Verification items for the finished model (mm, model axes). Face numbers are marked on the shaded views. A direction names the side the tool comes from. Round coordinates to 2 decimals unless told otherwise and drop trailing zeros. Order: outer loops, then holes, each group sorted by start corner. A loop starts at its lowest first (then second) coordinate and runs counter-clockwise, first axis right, second up. Notation, with made-up numbers: (-10, 87.25) -> (48, 87.25) arc R32 ccw to (48, 115.25) -> close; hole circle Ø10 at (5.5, 79). An arc over 180 degrees is marked (long way). Answer in a Markdown table with one row per item. Add a question column.
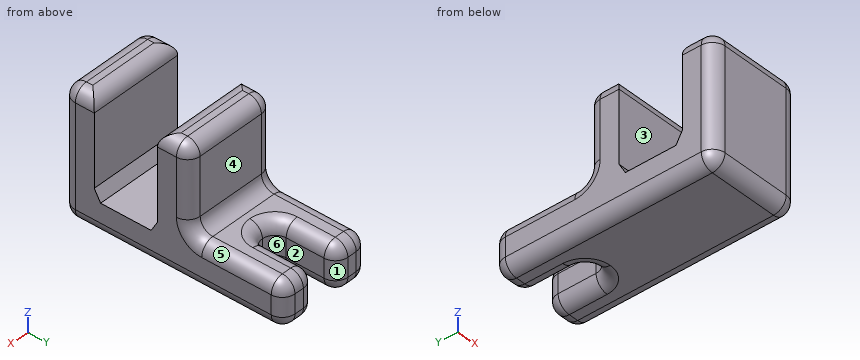
```python
from build123d import *

# Parameters (mm, degrees)
SKETCH1_W                      = 15
SKETCH1_H                      = 35
BOSS_EXTRUDE1_DEPTH            = 20
SKETCH2_W                      = 15
SKETCH2_H                      = 10
CUT_EXTRUDE1_DEPTH             = 44.011626335
SKETCH4_W                      = 13
SKETCH4_H                      = 15
CUT_EXTRUDE3_DEPTH             = 44.011626335
CUT_EXTRUDE4_REACH             = 45.012
SKETCH5_W                      = 4
SKETCH5_H                      = 10
CUT_EXTRUDE4_DIRECTION_2_DEPTH = 44.011626335
FILLET2_R                      = 2
CHAMFER1_SIZE                  = 1
CHAMFER1_SIZE2                 = 1.732050808


with BuildPart() as part:
    # Sketch1 → Boss-Extrude1 (new body)
    with BuildSketch(Plane.XY):
        with Locations((-7.5, 17.5)):
            Rectangle(SKETCH1_W, SKETCH1_H)
    extrude(amount=BOSS_EXTRUDE1_DEPTH)

    # Sketch2 → Cut-Extrude1 (cut, through all)
    with BuildSketch(Plane(origin=(0, 0, 0), x_dir=(0, 0, -1), z_dir=(1, 0, 0))):
        with Locations((-12.5, 10)):
            Rectangle(SKETCH2_W, SKETCH2_H)
    extrude(amount=-CUT_EXTRUDE1_DEPTH, mode=Mode.SUBTRACT)

    # Sketch4 → Cut-Extrude3 (cut, through all)
    with BuildSketch(Plane.ZY.offset(15)):
        with Locations((13.5, 27.5)):
            Rectangle(SKETCH4_W, SKETCH4_H)
    extrude(amount=-CUT_EXTRUDE3_DEPTH, mode=Mode.SUBTRACT)

    # Sketch5 → Cut-Extrude4 (cut, up to next)
    with BuildSketch(Plane(origin=(0, 0, 0), x_dir=(-1, 0, 0), z_dir=(0, 0, -1)), mode=Mode.PRIVATE) as cut_extrude4_sk1:
        with Locations((7.5, 30)):
            Rectangle(SKETCH5_W, SKETCH5_H)
    cut_extrude4_tool1 = extrude(cut_extrude4_sk1.sketch, amount=-CUT_EXTRUDE4_REACH, mode=Mode.PRIVATE) & part.part
    add(cut_extrude4_tool1.solids().sort_by_distance((-7.5, 30, 0))[0], mode=Mode.SUBTRACT)

    # Sketch5 → Cut-Extrude4 direction 2 (cut)
    with BuildSketch(Plane(origin=(0, 0, 0), x_dir=(-1, 0, 0), z_dir=(0, 0, -1))):
        with Locations((7.5, 30)):
            Rectangle(SKETCH5_W, SKETCH5_H)
    extrude(amount=CUT_EXTRUDE4_DIRECTION_2_DEPTH, mode=Mode.SUBTRACT)

    # Fillet2
    fillet2_edges = [part.edges().sort_by_distance(p)[0] for p in [
        (0, 17.5, 20),
        (-15, 2.5, 20),
        (-7.5, 0, 20),
        (-7.5, 5, 20),
        (-7.5, 15, 20),
        (-15, 17.5, 20),
        (-15, 35, 3.5),
        (0, 35, 3.5),
        (0, 20, 13.5),
        (-7.5, 20, 20),
        (0, 27.5, 7),
        (-7.5, 20, 7),
        (-2.75, 35, 7),
        (-15, 27.5, 7),
        (-15, 20, 13.5),
        (-12.25, 35, 7),
        (-12.25, 35, 0),
        (-5.5, 35, 3.5),
        (-5.5, 25, 3.5),
        (-9.5, 25, 3.5),
        (-9.5, 35, 3.5),
        (-5.5, 30, 0),
        (-7.5, 25, 0),
        (-9.5, 30, 0),
        (0, 2.5, 20),
        (-7.5, 0, 0),
        (-7.5, 25, 7),
        (-5.5, 30, 7),
        (-9.5, 30, 7),
        (-15, 17.5, 0),
        (-2.75, 35, 0),
        (0, 17.5, 0),
        (0, 0, 10),
        (-15, 0, 10),
    ]]
    fillet(fillet2_edges, radius=FILLET2_R - 0.0001)  # a hair under: the kernel refuses the full size

    # Chamfer1
    chamfer1_edges = [part.edges().sort_by_distance(p)[0] for p in [
        (-7.5, 15, 5),
        (-7.5, 5, 5),
    ]]
    chamfer1_side = [part.faces().sort_by_distance(p)[0] for p in [
        (-7.5, 10, 5),
    ]]
    chamfer(chamfer1_edges, length=CHAMFER1_SIZE, length2=CHAMFER1_SIZE2, reference=chamfer1_side[0])


solid = part.part
```
1) Cross-section at A-A, the plane z = 15.25. Record the boundary of the cut face in (x, y), and give its area (3 significant figures).
2) Thickness scan on L1, parallel to Y at x = -6, z = 13.5; L2, parallel to X at y = 29.5, z = 3.5; L3, parallel to Z at x = -3, y = 10.5. Record the ranges inside material, lowest first. Write a range as [from, to].
3) Depth check by flat-ended pin: P1, Ø7, axis at x = -5, z = 12, coming from the +Y side; P2, Ø1, axis at x = -4.5, z = 10, coming from the +Y side; P3, Ø2, axis at x = -10.5, y = 31, coming from the +Z side. Enter the tip coordinate at first touch or a pass-through.
4) Draft check along Y on the marked faces 1, 2 and 3. Enter one of: +Y half, -Y half, draft (parallel to the pull), parting line (faces both ways), or undercut.
5) Tool access check on the marked faces 4, 5 and 6. Record the directions out of +Z, -Z, +X, -X, +Y, -Y that give a thin tool (end or side, any length) a straight path to the whole face; none if there is none.
6) Cross-section at D-D, the plane y = 5.5. Record the boundary of the cut face in (x, z), and give its area (3 significant figures).
7) Cross-section at C-C, the plane y = 11. Record the boundary of the cut face in (x, z).
Results below:
| question | item | result |
|---|---|---|
| 1 | outline | (-15, 2) arc R2 ccw to (-13, 0) -> (-2, 0) arc R2 ccw to (0, 2) -> (0, 5) -> (-15, 5) -> close; (-15, 15) -> (0, 15) -> (0, 18) arc R2 ccw to (-2, 20) -> (-13, 20) arc R2 ccw to (-15, 18) -> close |
| 1 | area | 147 mm² |
| 2 | L1 | [0, 5], [15, 20] |
| 2 | L2 | [-15, -9.5], [-5.5, 0] |
| 2 | L3 | [0, 5] |
| 3 | P1 | y = 20.06 |
| 3 | P2 | y = 20 |
| 3 | P3 | z = 7 |
| 4 | face 1 | +Y half |
| 4 | face 2 | draft |
| 4 | face 3 | undercut |
| 5 | face 4 | +Z, +X, -X, +Y |
| 5 | face 5 | +Z, +X, +Y |
| 5 | face 6 | +Z, -Z, +Y |
| 6 | outline | (-15, 2) arc R2 ccw to (-13, 0) -> (-2, 0) arc R2 ccw to (0, 2) -> (0, 5.87) -> (-15, 5.87) -> close |
| 6 | area | 86.3 mm² |
| 7 | outline | (-15, 2) arc R2 ccw to (-13, 0) -> (-2, 0) arc R2 ccw to (0, 2) -> (0, 5) -> (-15, 5) -> close |
